```python
from build123d import *

# Parameters (mm, degrees)
BOSS_EXTRUDE1_DEPTH = 12.7
FILLET1_R           = 17.78
SKETCH2_R           = 7.9375
CUT_EXTRUDE1_DEPTH  = 25.4
SKETCH4_W           = 72.158320094
SKETCH4_H           = 56.919449397
CUT_EXTRUDE2_DEPTH  = 24.638
SKETCH5_R           = 2.032
CUT_EXTRUDE3_DEPTH  = 12.7
SKETCH6_R           = 4.1275
CUT_EXTRUDE4_DEPTH  = 32.258
SKETCH7_R           = 2.54
CUT_EXTRUDE5_DEPTH  = 12.7
FILLET2_R           = 2.54
SKETCH8_R           = 6.35
BOSS_EXTRUDE2_DEPTH = 12.7
SKETCH9_R           = 2.54
CUT_EXTRUDE6_DEPTH  = 12.7


with BuildPart() as part:
    # Sketch1 → Boss-Extrude1 (new body)
    with BuildSketch(Plane.XY):
        Polygon((-152.4, 0), (0, 0), (0, 152.4), align=None)
    extrude(amount=BOSS_EXTRUDE1_DEPTH)

    # Fillet1
    fillet1_edges = [part.edges().sort_by_distance(p)[0] for p in [
        (0, 152.4, 6.35),
    ]]
    fillet(fillet1_edges, radius=FILLET1_R)

    # Sketch2 → Cut-Extrude1 (cut)
    with BuildSketch(Plane.XY.offset(12.7)):
        with Locations((-16.51, 113.439359697)):
            Circle(SKETCH2_R)
        Polygon((-142.24, 0), (-152.4, 0), (-142.24, 10.16), align=None)
    extrude(amount=-CUT_EXTRUDE1_DEPTH, mode=Mode.SUBTRACT)

    # Sketch4 → Cut-Extrude2 (cut)
    with BuildSketch(Plane.XY):
        Polygon((-138.602769491, 5.715), (-114.068320094, 5.715), (-114.068320094, 30.249449397), align=None)
        Polygon((-110.258320094, 5.715), (-110.258320094, 34.059449397), (-81.683320094, 62.634449397), (-81.683320094, 5.715), align=None)
        Polygon((-77.873320094, 66.444449397), (-5.715, 66.444449397), (-5.715, 100.734449397), (-23.892955176, 100.734449397), (-32.002166338, 112.315603153), align=None)
        with Locations((-41.794160047, 34.174724699)):
            Rectangle(SKETCH4_W, SKETCH4_H)
    extrude(amount=CUT_EXTRUDE2_DEPTH, mode=Mode.SUBTRACT)

    # Sketch5 → Cut-Extrude3 (cut)
    with BuildSketch(Plane(origin=(0, 5.715, 0), x_dir=(1, 0, 0), z_dir=(0, 1, 0))):
        with Locations(Location((-126.365, -6.35, 0), (0, 0, 270))):
            Circle(SKETCH5_R)
    extrude(amount=-CUT_EXTRUDE3_DEPTH, mode=Mode.SUBTRACT)

    # Sketch6 → Cut-Extrude4 (cut)
    with BuildSketch(Plane(origin=(0, 5.715, 0), x_dir=(1, 0, 0), z_dir=(0, 1, 0))):
        with Locations(Location((-126.365, -6.35, 0), (0, 0, 180))):
            Circle(SKETCH6_R)
    extrude(amount=CUT_EXTRUDE4_DEPTH, mode=Mode.SUBTRACT)

    # Sketch7 → Cut-Extrude5 (cut)
    with BuildSketch(Plane(origin=(0, 5.715, 0), x_dir=(1, 0, 0), z_dir=(0, 1, 0))):
        with Locations(Location((-19.05, -6.35, 0), (0, 0, 270))):
            Circle(SKETCH7_R)
        with Locations(Location((-63.5, -6.35, 0), (0, 0, 270))):
            Circle(SKETCH7_R)
    extrude(amount=-CUT_EXTRUDE5_DEPTH, mode=Mode.SUBTRACT)

    # Fillet2
    fillet2_edges = [part.edges().sort_by_distance(p)[0] for p in [
        (-5.715, 5.715, 6.35),
    ]]
    fillet(fillet2_edges, radius=FILLET2_R)

    # Sketch8 → Boss-Extrude2 (add)
    with BuildSketch(Plane.XY.offset(12.7)):
        with Locations((-78.848031384, 63.088562946)):
            Circle(SKETCH8_R)
    extrude(amount=-BOSS_EXTRUDE2_DEPTH)

    # Sketch9 → Cut-Extrude6 (cut)
    with BuildSketch(Plane.XY.offset(12.7)):
        with Locations((-78.853278111, 63.331259387)):
            Circle(SKETCH9_R)
    extrude(amount=-CUT_EXTRUDE6_DEPTH, mode=Mode.SUBTRACT)


solid = part.part
```
CAD build for the part. Positions are in the model's coordinates, mm. A direction names the side the tool comes from. Round coordinates to 2 decimals unless told otherwise and drop trailing zeros. Loops run counter-clockwise (first coordinate to the right, second up) from the corner with the lowest first, then second, coordinate; pieces in that order, holes last. Notation, with made-up numbers: (-24, 54.25) - (-18, 54.25) arc R31 cw to (-18, 80.25) - close; hole circle Ø7 at (65.5, 87). An arc over 180 degrees is marked (long way). Return JSON: item names as keys, results as strings. Group by question number.
Q1. Band-saw the part on A-A on y = 82. Give the cut face in (x, z) (3 decimals), plus the area to 3 significant figures.
Q2. Tool access for faces 4 (the face through (-27.89, 106.44, 6.26)), 5 (the face through (-130.18, 21.96, 4.77)), 6 (the face through (-56, 64, 12.7)): list every direction of +Z, -Z, +X, -X, +Y, -Y with a clear straight run to the whole face (end or side of a thin tool).
Q3. Band-saw the part on B-B on x = -69. Give the cut face in (y, z) (3 decimals), plus the area to 3 significant figures.
Q4. Flat gauge pins, fed straight in: pin 1 Ø6.5 at (x, z) = (-130, 6) entering from +Y; pin 2 Ø5 at (y, z) = (36.5, 10.5) entering from -X; pin 3 Ø1.5 at (x, z) = (-43, 4.5) entering from +Y. Where does each tip first touch, or does it go through?
Q5. Drill centre lines: line 1 along X through (y, z) = (52, 6) (3 decimals); line 2 along Y through (x, z) = (-67, 4) (3 decimals); line 3 along X through (y, z) = (8.5, 7.25) (3 decimals). Where is each one in solid material? Low to high. Write a range as [from, to].
Q6. Two-plate mould, pull along Y, no slides. Class faces 1 (the face through (-17.54, 121.31, 6.44)), 2 (the face through (-85.5, 66.9, 6.3)), 3 (the face through (-16.53, 2.9, 6.02)): +Y half, -Y half, draft (parallel to the pull), parting line (faces both ways), or undercut.
Q7. Band-saw the part on D-D on z = 6.35. Give the number of separate pieces and of enclosed holes in the cut face, plus the area to 3 significant figures.
Q8. Band-saw the part on C-C on x = -19.05. Give the cut face in (y, z) (3 decimals), plus the area to 3 significant figures.
Solutions:
{
 "1": {"outline": "(-70.4, 0) - (-62.318, 0) - (-62.318, 12.7) - (-70.4, 12.7) - close; (-5.715, 0) - (0, 0) - (0, 12.7) - (-5.715, 12.7) - close", "area": "175 mm^2"},
 "2": {"face 4": "+Z, -Z", "face 5": "+Y", "face 6": "+Z, +X, -X, +Y, -Y"},
 "3": {"outline": "(0, 0) - (5.715, 0) - (5.715, 12.7) - (0, 12.7) - close; (62.634, 0) - (66.444, 0) - (66.444, 12.7) - (62.634, 12.7) - close; (75.318, 0) - (83.4, 0) - (83.4, 12.7) - (75.318, 12.7) - close", "area": "224 mm^2"},
 "4": {"pin 1": "stops at y = 23.63", "pin 2": "stops at x = -118.4", "pin 3": "stops at y = 110.15"},
 "5": {"line 1": "x = [-100.4, -92.318], [-81.683, -77.873], [-5.715, 0]", "line 2": "y = [0, 5.715], [62.634, 66.444], [77.318, 85.4]", "line 3": "x = [-142.24, -135.818], [-114.068, -110.258], [-81.683, -77.873], [-5.715, 0]"},
 "6": {"face 1": "undercut", "face 2": "+Y half", "face 3": "draft"},
 "7": {"separate pieces": "3", "enclosed holes": "4", "area": "3,210 mm^2"},
 "8": {"outline": "(0, 0) - (5.715, 0) - (5.715, 3.81) - (0, 3.81) - close; (0, 8.89) - (5.715, 8.89) - (5.715, 12.7) - (0, 12.7) - close; (62.634, 0) - (66.444, 0) - (66.444, 12.7) - (62.634, 12.7) - close; (100.734, 0) - (105.919, 0) - (105.919, 12.7) - (100.734, 12.7) - close; (120.959, 0) - (127.21, 0) - (127.21, 12.7) - (120.959, 12.7) - close", "area": "237 mm^2"}
}
